Check sheet for the modelled part. Datum: model origin and axes. Units: mm. A direction names the side the tool comes from. Round coordinates to 2 decimals unless told otherwise and drop trailing zeros. Write each loop counter-clockwise with the first axis right and the second up, starting at its lowest first coordinate (ties: lowest second). Pieces come first, ordered by that corner, then holes. Notation, with made-up numbers: (-38.75, -40) -> (-21.75, -40) arc R20 cw to (-21.75, -9) -> close; hole circle Ø6 at (-9, -31.75). An arc over 180 degrees is marked (long way). One line per item, written item: value.
from build123d import *

# Parameters (mm, degrees)
SKETCH1_W           = 160
SKETCH1_H           = 82
BOSS_EXTRUDE1_DEPTH = 10
SHELL1_T            = -2
SKETCH2_R           = 1
BOSS_EXTRUDE2_DEPTH = 16
FILLET1_R           = 2
FILLET2_R           = 2
FILLET3_R           = 2
FILLET4_R           = 2
SKETCH7_R           = 0.575
BOSS_EXTRUDE3_DEPTH = 6
SKETCH10_W          = 34
SKETCH10_H          = 8.029729716
CUT_EXTRUDE1_DEPTH  = 6
SKETCH16_W          = 80
SKETCH16_H          = 8
BOSS_EXTRUDE5_DEPTH = 5
SKETCH18_W          = 5
SKETCH18_H          = 8
BOSS_EXTRUDE6_DEPTH = 4
SKETCH21_W          = 63
SKETCH21_H          = 3
BOSS_EXTRUDE7_DEPTH = 0.9
SKETCH22_W          = 63
SKETCH22_H          = 3
BOSS_EXTRUDE8_DEPTH = 0.9


with BuildPart() as part:
    # Sketch1 → Boss-Extrude1 (new body)
    with BuildSketch(Plane(origin=(0, 0, 0), x_dir=(1, 0, 0), z_dir=(0, 1, 0))):
        Rectangle(SKETCH1_W, SKETCH1_H)
    extrude(amount=BOSS_EXTRUDE1_DEPTH)

    # Shell1
    shell1_openings = [part.faces().sort_by_distance(p)[0] for p in [
        (0, 10, 0),
    ]]
    offset(amount=SHELL1_T, openings=shell1_openings, kind=Kind.INTERSECTION)

    # Sketch2 → Boss-Extrude2 (add)
    with BuildSketch(Plane(origin=(0, 2, 0), x_dir=(1, 0, 0), z_dir=(0, 1, 0))):
        with Locations(Location((-75, 36, 0), (0, 0, 90))):
            Circle(SKETCH2_R)
        with Locations(Location((75, 36, 0), (0, 0, 90))):
            Circle(SKETCH2_R)
        with Locations(Location((75, -36, 0), (0, 0, 90))):
            Circle(SKETCH2_R)
        with Locations(Location((-75, -36, 0), (0, 0, 90))):
            Circle(SKETCH2_R)
    extrude(amount=BOSS_EXTRUDE2_DEPTH)

    # Fillet1
    fillet1_edges = [part.edges().sort_by_distance(p)[0] for p in [
        (-80, 5, 41),
    ]]
    fillet(fillet1_edges, radius=FILLET1_R)

    # Fillet2
    fillet2_edges = [part.edges().sort_by_distance(p)[0] for p in [
        (-80, 5, -41),
    ]]
    fillet(fillet2_edges, radius=FILLET2_R)

    # Fillet3
    fillet3_edges = [part.edges().sort_by_distance(p)[0] for p in [
        (80, 5, -41),
    ]]
    fillet(fillet3_edges, radius=FILLET3_R)

    # Fillet4
    fillet4_edges = [part.edges().sort_by_distance(p)[0] for p in [
        (80, 5, 41),
    ]]
    fillet(fillet4_edges, radius=FILLET4_R)

    # Sketch7 → Boss-Extrude3 (add)
    with BuildSketch(Plane(origin=(0, 2, 0), x_dir=(1, 0, 0), z_dir=(0, 1, 0))):
        with Locations(Location((-49, 24.45, 0), (0, 0, 90))):
            Circle(SKETCH7_R)
        with Locations(Location((-49, -24.43, 0), (0, 0, 90))):
            Circle(SKETCH7_R)
        with Locations(Location((8.9, -24.43, 0), (0, 0, 90))):
            Circle(SKETCH7_R)
        with Locations(Location((8.9, 24.45, 0), (0, 0, 90))):
            Circle(SKETCH7_R)
    extrude(amount=BOSS_EXTRUDE3_DEPTH)

    # Sketch10 → Cut-Extrude1 (cut)
    with BuildSketch(Plane.ZY.offset(80)):
        with Locations((7.4, 6.014864858)):
            Rectangle(SKETCH10_W, SKETCH10_H)
    extrude(amount=-CUT_EXTRUDE1_DEPTH, mode=Mode.SUBTRACT)

    # Sketch16 → Boss-Extrude5 (add)
    with BuildSketch(Plane(origin=(0, 2, 0), x_dir=(1, 0, 0), z_dir=(0, 1, 0))):
        with Locations((-32, 35)):
            Rectangle(SKETCH16_W, SKETCH16_H)
        with Locations((-32, -35)):
            Rectangle(SKETCH16_W, SKETCH16_H)
    extrude(amount=BOSS_EXTRUDE5_DEPTH)

    # Sketch18 → Boss-Extrude6 (add)
    with BuildSketch(Plane(origin=(0, 7, 0), x_dir=(1, 0, 0), z_dir=(0, 1, 0))):
        with Locations((-62.5, 35)):
            Rectangle(SKETCH18_W, SKETCH18_H)
        with Locations((5.5, 35)):
            Rectangle(SKETCH18_W, SKETCH18_H)
        with Locations((5.5, -35)):
            Rectangle(SKETCH18_W, SKETCH18_H)
        with Locations((-62.5, -35)):
            Rectangle(SKETCH18_W, SKETCH18_H)
    extrude(amount=BOSS_EXTRUDE6_DEPTH)

    # Sketch21 → Boss-Extrude7 (add)
    with BuildSketch(Plane.XY.offset(-39)):
        with Locations((-28.5, 8.5)):
            Rectangle(SKETCH21_W, SKETCH21_H)
    extrude(amount=BOSS_EXTRUDE7_DEPTH)

    # Sketch22 → Boss-Extrude8 (add)
    with BuildSketch(Plane(origin=(0, 0, 39), x_dir=(-1, 0, 0), z_dir=(0, 0, -1))):
        with Locations((28.5, 8.5)):
            Rectangle(SKETCH22_W, SKETCH22_H)
    extrude(amount=BOSS_EXTRUDE8_DEPTH)


solid = part.part
Item 1: Tool access check on faces 1 (the flat face through (-33, 4, 31)), 2 (the flat face through (-63, 11, -35)). Record the directions out of +Z, -Z, +X, -X, +Y, -Y that give a thin tool (end or side, any length) a straight path to the whole face; none if there is none.
Result set:
face 1: +Y
face 2: +Z, -Z, +Y
Item 2: Sectioned sample at D-D (y = 14.75). Enter the section's corners in (x, z).
Result set:
outline: circle Ø2 at (-75, -36); circle Ø2 at (-75, 36); circle Ø2 at (75, -36); circle Ø2 at (75, 36)
Item 3: Depth check by flat-ended pin: pin 1 (3 mm diameter, centred on x = -61, z = -19.5, fed in from +Y); pin 2 (8 mm diameter, centred on y = 14.5, z = -21, fed in from +X); pin 3 (1.3 mm diameter, centred on x = -49, z = 24.5, fed in from +Y); pin 4 (5.5 mm diameter, centred on x = 6.5, z = 37, fed in from +Y). Enter the tip coordinate at first touch or a pass-through.
Result set:
pin 1: y = 2
pin 2: through
pin 3: y = 8
pin 4: y = 11
Item 4: Sectioned sample at B-B (x = -63.5). Enter the section's corners in (y, z).
Result set:
outline: (0, -41) -> (10, -41) -> (10, -39) -> (11, -39) -> (11, -31) -> (2, -31) -> (2, 31) -> (11, 31) -> (11, 39) -> (10, 39) -> (10, 41) -> (0, 41) -> close
Item 5: Sectioned sample at A-A (y = 5.25). State how many separate pieces and enclosed holes the cut face has, then the cut area to 3 significant figures.
Result set:
separate pieces: 9
enclosed holes: 0
area: 2,180 mm^2
Item 6: Material ranges on line 1 along Z through (x, y) = (-59.5, 9.5); line 2 along X through (y, z) = (6.25, 24); line 3 along X through (y, z) = (8.5, 29), recorded low to high.
Result set:
line 1: -41 to -38.1, 38.1 to 41
line 2: -49.38 to -48.62, 8.52 to 9.28, 78 to 80
line 3: -80 to -78, 78 to 80
Item 7: Release check for a two-part mould opening along X. For faces 3 (the flat face through (-1, 5, 41)), 4 (the flat face through (-80, 1.6, 0.5)), 5 (the flat face through (8, 6, -35)) record: pulls with the +X half, pulls with the -X half, needs draft (parallel to the pull), parting line crosses it, or undercut.
Result set:
face 3: needs draft
face 4: pulls with the -X half
face 5: undercut
Item 8: Sectioned sample at C-C (z = 28). Enter the section's corners in (x, y), then the cut area to 3 significant figures.
Result set:
outline: (-80, 0) -> (80, 0) -> (80, 10) -> (78, 10) -> (78, 2) -> (-78, 2) -> (-78, 10) -> (-80, 10) -> close
area: 352 mm^2
